Verification items for the finished model (mm, model axes). A direction names the side the tool comes from. Give positions to 0.01 mm unless a question says otherwise; leave off trailing zeros. Order: outer loops, then holes, each group sorted by start corner. A loop starts at its lowest first (then second) coordinate and runs counter-clockwise, first axis right, second up. Notation, with made-up numbers: (48.25, -35.5) - (99.25, -35.5) arc R13 ccw to (99.25, -15.5) - close; hole circle Ø11 at (-7, 54.25). An arc over 180 degrees is marked (long way). Answer as a JSON object with one key per item and string values.
Autodesk Inventor part; units mm, degrees
ref_plane "YZ Plane" through (0, 0, 0) normal (1, 0, 0) x (0, 1, 0)
ref_plane "XZ Plane" through (0, 0, 0) normal (0, 1, 0) x (-1, 0, 0)
ref_plane "XY Plane" through (0, 0, 0) normal (0, 0, 1) x (1, 0, 0)
sketch "Sketch1" plane through (0, 0, 0) normal (0, 1, 0) x (-1, 0, 0)
  line L0 (10, -15.715) -> (-10, -15.715)
  line L1 (-10, -15.715) -> (-10, 15.715)
  line L2 (-10, 15.715) -> (10, 15.715)
  line L3 (10, 15.715) -> (10, -15.715)
  point P0 (0, 0)
  dimension "d0" = 20
  dimension "d1" = 31.43
  dimension "d2" = 10
  dimension "d3" = 15.715
extrude "Plate1" add sketch "Sketch1" along normal blind 1.5
sketch "Sketch2" plane through (10, 0, 17.215) normal (0, 0, -1) x (-1, 0, 0)
  line L0 (20, 0) -> (0, 0)
  line L1 (0, 0) -> (0, 40)
  line L2 (0, 40) -> (20, 40)
  line L3 (20, 40) -> (20, 0)
edge flange "Flange1" height 40 angle 90 thickness 1.5 bend radius 0.31 thickness toward (0, 0, -1) relief tear relief width 1.5 relief depth 0.75 edges at (0, 1.5, 15.715) wall of the first edge with corners at (-10, 0, 17.215) (10, 0, 17.215) (10, 40, 17.215) (-10, 40, 17.215)
bend "Bend1"
corner "Corner1"
sketch "Sketch3" plane through (-10, 0, -17.215) normal (0, 0, 1) x (1, 0, 0)
  line L0 (20, 0) -> (0, 0)
  line L1 (0, 0) -> (0, 40)
  line L2 (0, 40) -> (20, 40)
  line L3 (20, 40) -> (20, 0)
edge flange "Flange2" height 40 angle 90 thickness 1.5 bend radius 0.31 thickness toward (0, 0, 1) relief tear relief width 1.5 relief depth 0.75 edges at (0, 1.5, -15.715) wall of the first edge with corners at (10, 0, -17.215) (-10, 0, -17.215) (-10, 40, -17.215) (10, 40, -17.215)
bend "Bend2"
corner "Corner2"
equation "\"d4\" = Thickness"
equation "\"d5\" = BendReliefWidth"
equation "\"d6\" = BendReliefDepth"
equation "\"d7\" = MinimumRemnant"
equation "\"d8\" = TransitionRadius"
equation "\"d11\" = BendRadius"
equation "\"d12\" = CornerReliefSize"
equation "\"d13\" = GapSize"
equation "\"d14\" = JacobiRadiusSize"
equation "\"d15\" = BendReliefWidth"
equation "\"d16\" = BendReliefDepth"
equation "\"d17\" = MinimumRemnant"
equation "\"d18\" = TransitionRadius"
equation "\"d21\" = BendRadius"
equation "\"d22\" = CornerReliefSize"
equation "\"d23\" = GapSize"
equation "\"d24\" = JacobiRadiusSize"
equation "\"BendReliefWidth\" = Thickness"
equation "\"BendReliefDepth\" = 0.5 * Thickness"
equation "\"CornerReliefSize\" = 4 * Thickness"
equation "\"MinimumRemnant\" = 2 * Thickness"
equation "\"TransitionRadius\" = BendRadius"
equation "\"JacobiRadiusSize\" = BendRadius"
equation "\"GapSize\" = Thickness"
properties part number "axis_7_top_frame" material "Aluminum 6061-AHC"
(1) Section check A-A (y = 14.5). Record the cut outline in (x, z) (3 decimals).
Computed values:
{"outline": "(-10, -17.215) - (10, -17.215) - (10, -15.715) - (-10, -15.715) - close; (-10, 15.715) - (10, 15.715) - (10, 17.215) - (-10, 17.215) - close"}
(2) Release check for a two-part mould opening along Z. For faces 3 (the flat face through (0, 1.5, 0)), 4 (the cylindrical face through (-0.14, 0.544, -16.699)), 5 (the flat face through (0, 21, 15.715)), 6 (the flat face through (-10, 1, 0)) record: pulls with the +Z half, pulls with the -Z half, needs draft (parallel to the pull), parting line crosses it, or undercut.
Computed values:
{"face 3": "undercut", "face 4": "pulls with the -Z half", "face 5": "undercut", "face 6": "needs draft"}
(3) Access from +Z, -Z, +X, -X, +Y, -Y to the whole of each face (thin tool, end or side, straight path). Record for faces 1 (the flat face through (10, 1, 0)), 2 (the flat face through (0, 21, -15.715)).
Computed values:
{"face 1": "+Z, -Z, +X, +Y, -Y", "face 2": "+X, -X, +Y"}
(4) Section check B-B (x = -2.75). Record the cut outline in (y, z) (3 decimals).
Computed values:
{"outline": "(0, -15.405) arc R1.81 ccw to (1.81, -17.215) - (40, -17.215) - (40, -15.715) - (1.81, -15.715) arc R0.31 cw to (1.5, -15.405) - (1.5, 15.405) arc R0.31 cw to (1.81, 15.715) - (40, 15.715) - (40, 17.215) - (1.81, 17.215) arc R1.81 ccw to (0, 15.405) - close"}
(5) Gauge pin test, flat ends, axial feed: pin 1 Ø1 at (x, z) = (0, -9) entering from -Y; pin 2 Ø4 at (x, z) = (5, -13.5) entering from +Y. Record the tip position at first contact, or that the pin passes through.
Computed values:
{"pin 1": "stops at y = 0", "pin 2": "stops at y = 1.51"}
(6) Material ranges on line 1 along Z through (x, y) = (9.25, 11.5) (3 decimals); line 2 along Y through (x, z) = (1, -15), recorded low to high. Write a range as [from, to].
Computed values:
{"line 1": "z = [-17.215, -15.715], [15.715, 17.215]", "line 2": "y = [0, 1.5]"}
(7) Section check C-C (z = -13.5). Record the cut outline in (x, y).
Computed values:
{"outline": "(-10, 0) - (10, 0) - (10, 1.5) - (-10, 1.5) - close"}
